from build123d import *

# Parameters (mm, degrees)
F0_W     = 67
F0_H     = 131.1
F1_DEPTH = 6.9
F2_R     = 3
F3_R     = 5.65049
F4_DEPTH = 2
F5_R     = 1
F7_DEPTH = 1
F8_R     = 5


with BuildPart() as f1:
    # F0 (on Top) → F1 (new body)
    with BuildSketch(Plane.XY):
        with Locations((-19.632723, -10.392761)):
            Rectangle(F0_W, F0_H)
    extrude(amount=F1_DEPTH)

    # F2
    f2_edges = [f1.edges().sort_by_distance(p)[0] for p in [
        (-19.632723, 55.157239, 6.9),
        (-53.132723, -10.392761, 6.9),
        (-19.632723, -75.942761, 6.9),
        (13.867277, -10.392761, 6.9),
        (-19.632723, 55.157239, 0),
        (-53.132723, -10.392761, 0),
        (-19.632723, -75.942761, 0),
        (13.867277, -10.392761, 0),
        (13.867277, -75.942761, 3.45),
        (-53.132723, -75.942761, 3.45),
        (13.867277, 55.157239, 3.45),
        (-53.132723, 55.157239, 3.45),
    ]]
    fillet(f2_edges, radius=F2_R)

    # F3 (on face) → F4 (cut)
    with BuildSketch(Plane.XY.offset(6.9)):
        with Locations((-19.632723, -63.500725)):
            Circle(F3_R)
        Polygon((-11.632723, 48.157239), (-19.632723, 48.157239), (-27.632723, 48.157239), (-27.632723, 45.157239), (-11.632723, 45.157239), align=None)
    extrude(amount=-F4_DEPTH, mode=Mode.SUBTRACT)

    # F5
    f5_edges = [f1.edges().sort_by_distance(p)[0] for p in [
        (-27.632723, 45.157239, 5.9),
        (-27.632723, 48.157239, 5.9),
        (-11.632723, 48.157239, 5.9),
        (-11.632723, 45.157239, 5.9),
    ]]
    fillet(f5_edges, radius=F5_R)

    # F6 (on face) → F7 (cut)
    with BuildSketch(Plane.XY.offset(6.9)):
        Polygon((-48.132723, 50.157239), (-48.132723, 49.157239), (-48.132723, -70.942761), (8.867277, -70.942761), (8.867277, 50.157239), align=None)
    extrude(amount=-F7_DEPTH, mode=Mode.SUBTRACT)

    # F8
    f8_edges = [f1.edges().sort_by_distance(p)[0] for p in [
        (-48.132723, 50.157239, 6.4),
        (8.867277, 50.157239, 6.4),
        (8.867277, -70.942761, 6.4),
        (-48.132723, -70.942761, 6.4),
    ]]
    fillet(f8_edges, radius=F8_R)


solid = f1.part
Design review of the part built by this model. Coordinates are the model's own, in mm. A direction names the side the tool comes from. Round coordinates to 2 decimals unless told otherwise and drop trailing zeros. Order: outer loops, then holes, each group sorted by start corner. A loop starts at its lowest first (then second) coordinate and runs counter-clockwise, first axis right, second up. Notation, with made-up numbers: M -8.5,58 L 38.5,58 A15 ccw 38.5,86 Z; hole C 22,18.5 d2. An arc over 180 degrees is marked long. Answer as CSV lines item,"result". Start each with the question number.
1) The part is to be moulded in two halves that separate along Y. For faces 3 (the face through (-19.2, 54.3, 0.9)), 4 (the face through (-20, 47, 4.9)), 5 (the face through (-52.277, -9.517, 0.902)), say which applies: +Y half, -Y half, draft (parallel to the pull), parting line (faces both ways), or undercut.
2) Wall thickness on line 1 along Z through (x, y) = (-10.5, 37.5); line 2 along Y through (x, z) = (-23.5, 5); line 3 along Y through (x, z) = (-17, 4.25): over which ranges is each line inside the solid? List them lowest first. Write a range as [from, to].
3) Add section B-B (y = 28). Give the boundary of the cut face in (x, z), then the cut area to 3 significant figures.
4) For pin 1 Ø2.5 at (x, y) = (-23, 46.5) entering from +Z; pin 2 Ø0.5 at (y, z) = (46.5, 5) entering from -X; pin 3 Ø1.5 at (y, z) = (-51.5, 0.5) entering from +X, all flat-tipped, find the tip position at first contact; note any pin that passes through.
5) Add section A-A (x = -9). Give the boundary of the cut face in (y, z), then the cut area to 3 significant figures.
6) Add section C-C (z = 1.5). Give the boundary of the cut face in (x, y), then the cut area to 3 significant figures.
7) Tool access review of faces 1 (the face through (-20, -10, 0)), 2 (the face through (-20, -10, 5.9)): name each direction out of +Z, -Z, +X, -X, +Y, -Y from which nothing blocks a thin tool from reaching the whole face with its end or side.
Resolved:
1,face 3,"+Y half"
1,face 4,"undercut"
1,face 5,"draft"
2,line 1,"[0, 5.9]"
2,line 2,"[-75.73, -67.62], [-59.38, 45.16], [48.16, 54.95]"
2,line 3,"[-75.92, 55.14]"
3,outline,"M -53.13,3 A3 ccw -50.13,0 L 10.87,0 A3 ccw 13.87,3 L 13.87,3.9 A3 ccw 10.87,6.9 L 8.87,6.9 L 8.87,5.9 L -48.13,5.9 L -48.13,6.9 L -50.13,6.9 A3 ccw -53.13,3.9 Z"
3,area,"398 mm^2"
4,pin 1,"z = 4.9"
4,pin 2,"x = -53.01"
4,pin 3,"x = 13.3"
5,outline,"M -75.94,3 A3 ccw -72.94,0 L 52.16,0 A3 ccw 55.16,3 L 55.16,3.9 A3 ccw 52.16,6.9 L 50.16,6.9 L 50.16,5.9 L -70.94,5.9 L -70.94,6.9 L -72.94,6.9 A3 ccw -75.94,3.9 Z"
5,area,"776 mm^2"
6,outline,"M -52.73,-72.94 A2.6 ccw -50.13,-75.54 L 10.87,-75.54 A2.6 ccw 13.47,-72.94 L 13.47,52.16 A2.6 ccw 10.87,54.76 L -50.13,54.76 A2.6 ccw -52.73,52.16 Z"
6,area,"8,620 mm^2"
7,face 1,"-Z, +X, -X, +Y, -Y"
7,face 2,"+Z"
